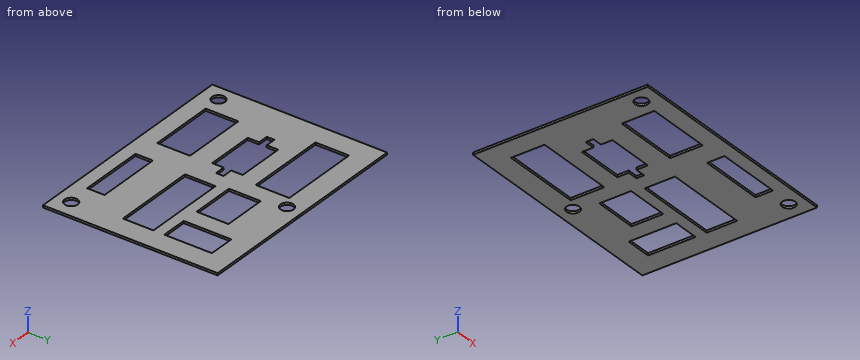
Autodesk Inventor part; units mm, degrees
ref_plane "YZ Plane" through (0, 0, 0) normal (1, 0, 0) x (0, 1, 0)
ref_plane "XZ Plane" through (0, 0, 0) normal (0, 1, 0) x (-1, 0, 0)
ref_plane "XY Plane" through (0, 0, 0) normal (0, 0, 1) x (1, 0, 0)
sketch "Sketch1" plane through (0, 0, 0) normal (0, 0, 1) x (1, 0, 0)
  line L0 (-52.5, 40) -> (52.5, 40)
  line L1 (52.5, 40) -> (52.5, -40)
  line L2 (52.5, -40) -> (-52.5, -40)
  line L3 (-52.5, -40) -> (-52.5, 40)
  line L4 (-52.5, 40) -> (52.5, -40) construction
  line L5 (52.5, 40) -> (-52.5, -40) construction
  point P0 (0, 0)
  dimension "d0" = 80
  dimension "d1" = 105
extrude "Plate1" add sketch "Sketch1" along normal blind 1
sketch "Sketch3" plane through (0, 0, 0) normal (0, 0, -1) x (-1, 0, 0)
  line L0 (-42.5, 3.2) -> (-4, 3.2)
  line L1 (-4, 3.2) -> (-4, -10.8)
  line L2 (-4, -10.8) -> (-42.5, -10.8)
  line L3 (-42.5, -10.8) -> (-42.5, 3.2)
  line L4 (-42.5, 3.2) -> (-4, -10.8) construction
  line L5 (-4, 3.2) -> (-42.5, -10.8) construction
  line L6 (8.25, 6.6) -> (30.25, 6.6)
  line L7 (35, 1.35) -> (35, -2.15)
  line L8 (30.25, -7.4) -> (8.25, -7.4)
  line L9 (3.5, -2.15) -> (3.5, 1.35)
  line L10 (0.2073, 10) -> (38.2927, -10.8) construction
  line L11 (35, 6.6) -> (3.5, -7.4) construction
  line L12 (-2.5, 8.2) -> (-22.5, 8.2)
  line L13 (-22.5, 8.2) -> (-22.5, 22.8)
  line L14 (-22.5, 22.8) -> (-2.5, 22.8)
  line L15 (-2.5, 22.8) -> (-2.5, 8.2)
  line L16 (-2.5, 8.2) -> (-22.5, 22.8) construction
  line L17 (-22.5, 8.2) -> (-2.5, 22.8) construction
  line L18 (-3.29, -34) -> (-33.29, -34)
  line L19 (-33.29, -34) -> (-33.29, -26)
  line L20 (-33.29, -26) -> (-3.29, -26)
  line L21 (-3.29, -26) -> (-3.29, -34)
  line L22 (-3.29, -34) -> (-33.29, -26) construction
  line L23 (-33.29, -34) -> (-3.29, -26) construction
  line L24 (52.5, 40) -> (-52.5, 40)
  line L25 (52.5, -40) -> (52.5, 40)
  line L26 (30.25, -7.4) -> (30.25, -2.15)
  line L27 (30.25, -2.15) -> (35, -2.15)
  line L28 (30.25, 6.6) -> (30.25, 1.35)
  line L29 (30.25, 1.35) -> (35, 1.35)
  line L30 (8.25, -7.4) -> (8.25, -2.15)
  line L31 (8.25, -2.15) -> (3.5, -2.15)
  line L32 (8.25, 6.6) -> (8.25, 1.35)
  line L33 (8.25, 1.35) -> (3.5, 1.35)
  line L34 (-52.5, 40) -> (-52.5, -40)
  line L35 (-42.5, 30) -> (-30.5, 30)
  line L36 (-30.5, 30) -> (-30.5, 8.2)
  line L37 (-30.5, 8.2) -> (-42.5, 8.2)
  line L38 (-42.5, 8.2) -> (-42.5, 30)
  line L39 (7.5, -32) -> (37.5, -32)
  line L40 (37.5, -32) -> (37.5, -17)
  line L41 (37.5, -17) -> (7.5, -17)
  line L42 (7.5, -17) -> (7.5, -32)
  line L43 (-52.5, -40) -> (52.5, -40)
  point P0 (0, 0)
  point P1 (-23.25, -3.8)
  point P2 (19.25, -0.4)
  point P3 (-12.5, 15.5)
  point P4 (-18.29, -30)
  dimension "d14" = 14
  dimension "d17" = 7.5
  dimension "d22" = 20
  dimension "d24" = 14.6
  dimension "d37" = 8
  dimension "d40" = 30
  dimension "d46" = 17.2
  dimension "d47" = 55
  dimension "d48" = 17.5
  dimension "d49" = 33.4
  dimension "d50" = 66
  dimension "d65" = 14
  dimension "d66" = 31.5
  dimension "d67" = 3.5
  dimension "d68" = 22
  dimension "d69" = 5
  dimension "d70" = 10
  dimension "d71" = 10
  dimension "d72" = 10
  dimension "d73" = 8
  dimension "d74" = 5
  dimension "d75" = 19.21
  dimension "d76" = 15
  dimension "d77" = 8
  dimension "d78" = 15
  dimension "d79" = 30
extrude "Extrusion1" cut sketch "Sketch3" against normal blind 10 contours L0 L1 L2 L3 | L6 L28 L29 L7 L27 L26 L8 L30 L31 L9 L33 L32 | L12 L13 L14 L15 | L18 L19 L20 L21 | L35 L36 L37 L38 | L42 L41 L40 L39
sketch "Sketch5" plane through (0, 0, 0) normal (0, 0, -1) x (-1, 0, 0)
  line L0 (42.5, 14.6) -> (5.5, 14.6)
  line L1 (5.5, 14.6) -> (5.5, 30)
  line L2 (5.5, 30) -> (42.5, 30)
  line L3 (42.5, 30) -> (42.5, 14.6)
  line L4 (42.5, 14.6) -> (5.5, 30) construction
  line L5 (5.5, 14.6) -> (42.5, 30) construction
  line L6 (8.25, 6.6) -> (30.25, 6.6)
  line L7 (-2.5, 22.8) -> (-2.5, 8.2)
  line L8 (-4, -10.8) -> (-42.5, -10.8)
  line L9 (52.5, 40) -> (-52.5, 40)
  line L10 (52.5, -40) -> (52.5, 40)
  point P0 (0, 0)
  point P1 (24, 22.3)
  point P2 (3.5, 1.6)
  point P3 (35, 1.6)
  point P4 (24, 14.6)
  dimension "d27" = 8
  dimension "d28" = 8
  dimension "d52" = 10
  dimension "d53" = 10
extrude "Extrusion2" cut sketch "Sketch5" against normal blind 10
sketch "Sketch7" plane through (0, 0, 0) normal (0, 0, -1) x (-1, 0, 0)
  point P0 (0, 0)
sketch "Sketch8" plane through (0, 0, 0) normal (0, 0, -1) x (-1, 0, 0)
  circle A0 centre (45.5, -32) radius 3
  circle A1 centre (-44.5, -33) radius 3
  circle A2 centre (0, 33) radius 3
  line L0 (52.5, -40) -> (52.5, 40)
  line L1 (-52.5, -40) -> (52.5, -40)
  line L2 (-52.5, 40) -> (-52.5, -40)
  line L3 (52.5, 40) -> (-52.5, 40)
  point P0 (0, 0)
  dimension "d54" = 6
  dimension "d55" = 6
  dimension "d56" = 6
  dimension "d57" = 7
  dimension "d58" = 8
  dimension "d60" = 8
  dimension "d61" = 7
  dimension "d62" = 7
extrude "Extrusion3" cut sketch "Sketch8" against normal blind 10 contours A0 | A1 | A2
equation "\"d2\" = 厚度"
equation "\"折彎半徑\" = 厚度"
equation "\"最小剩餘\" = 2 * 厚度"
equation "\"轉移半徑\" = 折彎半徑"
equation "\"間隙大小\" = 厚度"
equation "\"折彎離隙寬度\" = 厚度"
equation "\"折彎離隙深度\" = 0.5 * 厚度"
equation "\"轉角離隙大小\" = 4 * 厚度"
equation "\"Jacobi半徑大小\" = 折彎半徑"
properties part number "cap"
Geometry check sheet. Reference: the model listing, model coordinates, mm. Give positions to 0.01 mm unless a question says otherwise; leave off trailing zeros. Order: outer loops, then holes, each group sorted by start corner. A loop starts at its lowest first (then second) coordinate and runs counter-clockwise, first axis right, second up. Notation, with made-up numbers: (45, 48.25) - (59, 48.25) arc R17 cw to (59, 73.25) - close; hole circle Ø2 at (-13.5, -40). An arc over 180 degrees is marked (long way). Answer in a Markdown table with one row per item. Add a question column.
Q1. Cross-section at A-A, the plane y = 33. Enter the section's corners in (x, z), then the cut area to 3 significant figures.
Q2. Material ranges on probe 1 along X at (y, z) = (27, 0.5); probe 2 along Y at (x, z) = (-19, 0.2); probe 3 along Y at (x, z) = (22, 0.95), recorded low to high. Write a range as from..to.
Q3. Cross-section at D-D, the plane x = -45.5. Enter the section's corners in (y, z).
Q4. Cross-section at C-C, the plane x = 8.5. Enter the section's corners in (y, z).
Q5. Cross-section at B-B, the plane y = 21.5. Enter the section's corners in (x, z), then the cut area to 3 significant figures.
Check values:
| question | item | result |
|---|---|---|
| 1 | outline | (-52.5, 0) - (-3, 0) - (-3, 1) - (-52.5, 1) - close; (3, 0) - (52.5, 0) - (52.5, 1) - (3, 1) - close |
| 1 | area | 99.0 mm^2 |
| 2 | probe 1 | x = -52.5..-42.5, -5.5..30.5, 42.5..52.5 |
| 2 | probe 2 | y = -40..-32, -17..-7.4, 6.6..14.6, 30..40 |
| 2 | probe 3 | y = -40..-34, -26..-10.8, 3.2..8.2, 22.8..40 |
| 3 | outline | (-40, 0) - (-35, 0) - (-35, 1) - (-40, 1) - close; (-29, 0) - (40, 0) - (40, 1) - (-29, 1) - close |
| 4 | outline | (-40, 0) - (-34, 0) - (-34, 1) - (-40, 1) - close; (-26, 0) - (-10.8, 0) - (-10.8, 1) - (-26, 1) - close; (3.2, 0) - (8.2, 0) - (8.2, 1) - (3.2, 1) - close; (22.8, 0) - (40, 0) - (40, 1) - (22.8, 1) - close |
| 5 | outline | (-52.5, 0) - (-42.5, 0) - (-42.5, 1) - (-52.5, 1) - close; (-5.5, 0) - (2.5, 0) - (2.5, 1) - (-5.5, 1) - close; (22.5, 0) - (30.5, 0) - (30.5, 1) - (22.5, 1) - close; (42.5, 0) - (52.5, 0) - (52.5, 1) - (42.5, 1) - close |
| 5 | area | 36.0 mm^2 |
